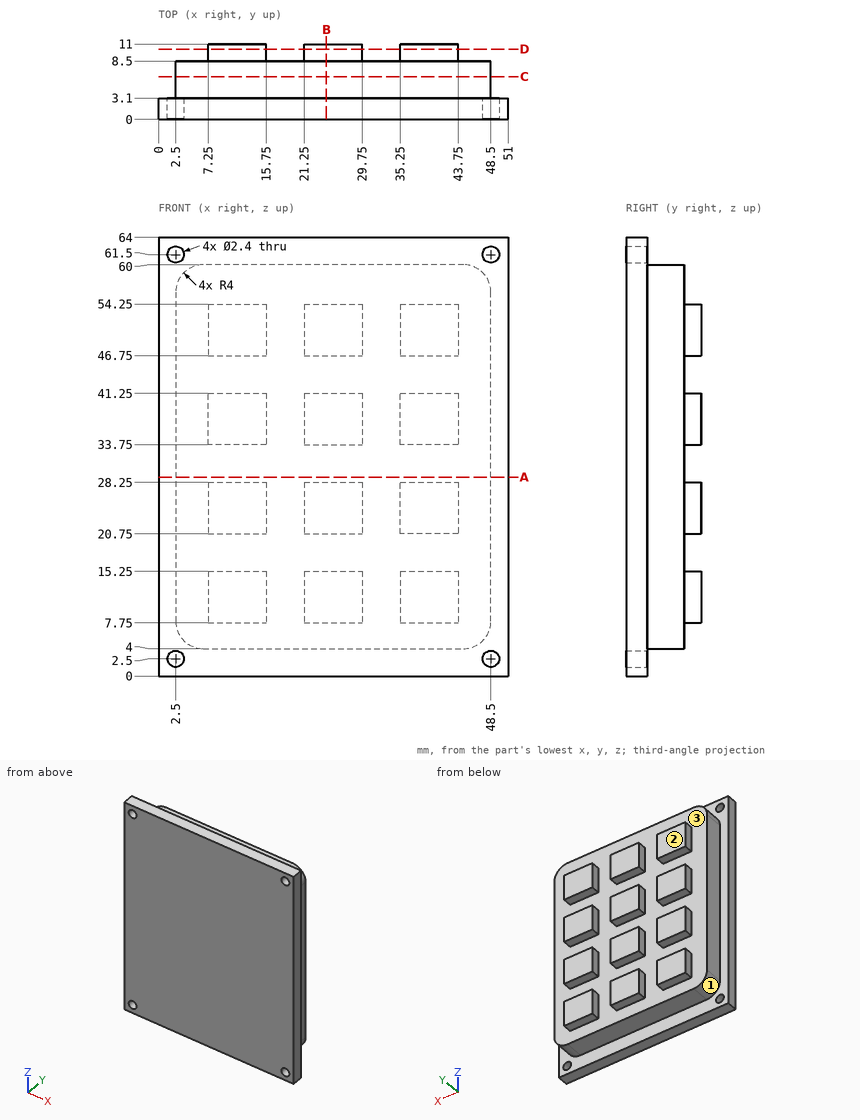
Input: dimensioned drawing with shaded views. Units: mm. Origin: part minimum x, y, z. Coordinates: 2 decimals unless noted, no trailing zeros. Loops run counter-clockwise (first coordinate to the right, second up) from the corner with the lowest first, then second, coordinate; pieces in that order, holes last. Notation, with made-up numbers: M 16.25,-8 L 24.25,-8 A24 ccw 24.25,3 Z; hole C -39.5,61.25 d10. An arc over 180 degrees is marked long. Use a Markdown table: item, result. Add a question column.
Q1. Section query A-A, the plane z = 29. Return loops of the section in (x, y), and give its area (4 significant figures).
Q2. First-contact query: pin 1 (0.8 mm diameter, centred on y = 10, z = 36, fed in from -X); pin 2 (0.8 mm diameter, centred on x = 27.5, y = 10, fed in from -Z); pin 3 (3 mm diameter, centred on y = 9.5, z = 12, fed in from -X). Flat tips, straight axial feed; report the tip coordinate or a pass-through.
Q3. Section query C-C, the plane y = 6.25. Return loops of the section in (x, z).
Q4. Material intervals for L1, parallel to X at y = 1.5, z = 61.5; L2, parallel to Z at x = 29.5, y = 9.5; L3, parallel to Z at x = 48.5, y = 1.4, sorted ascending.
Q5. Section query D-D, the plane y = 10.25. State how many separate pieces and enclosed holes the cut face has, and give its area (3 significant figures).
Q6. Draft query along Z for the marked faces 1, 2 and 3. Return one class per face: pulls with the +Z half, pulls with the -Z half, needs draft (parallel to the pull), parting line crosses it, or undercut.
Q7. Section query B-B, the plane x = 24.5. Return loops of the section in (y, z).
Result:
| question | item | result |
|---|---|---|
| 1 | outline | M 0,0 L 51,0 L 51,3.1 L 48.5,3.1 L 48.5,8.5 L 2.5,8.5 L 2.5,3.1 L 0,3.1 Z |
| 1 | area | 406.5 mm2 |
| 2 | pin 1 | stops at x = 7.25 |
| 2 | pin 2 | stops at z = 7.75 |
| 2 | pin 3 | stops at x = 2.5 |
| 3 | outline | M 2.5,8 A4 ccw 6.5,4 L 44.5,4 A4 ccw 48.5,8 L 48.5,56 A4 ccw 44.5,60 L 6.5,60 A4 ccw 2.5,56 Z |
| 4 | L1 | x = 0 to 1.3, 3.7 to 47.3, 49.7 to 51 |
| 4 | L2 | z = 7.75 to 15.25, 20.75 to 28.25, 33.75 to 41.25, 46.75 to 54.25 |
| 4 | L3 | z = 0 to 1.3, 3.7 to 60.3, 62.7 to 64 |
| 5 | separate pieces | 12 |
| 5 | enclosed holes | 0 |
| 5 | area | 765 mm2 |
| 6 | face 1 | pulls with the -Z half |
| 6 | face 2 | needs draft |
| 6 | face 3 | undercut |
| 7 | outline | M 0,0 L 3.1,0 L 3.1,4 L 8.5,4 L 8.5,7.75 L 11,7.75 L 11,15.25 L 8.5,15.25 L 8.5,20.75 L 11,20.75 L 11,28.25 L 8.5,28.25 L 8.5,33.75 L 11,33.75 L 11,41.25 L 8.5,41.25 L 8.5,46.75 L 11,46.75 L 11,54.25 L 8.5,54.25 L 8.5,60 L 3.1,60 L 3.1,64 L 0,64 Z |
